Part print with two shaded views. Sizes in mm from the minimum x, y, z corner. Coordinates: 2 decimals unless noted, no trailing zeros. Write each loop counter-clockwise with the first axis right and the second up, starting at its lowest first coordinate (ties: lowest second). Pieces come first, ordered by that corner, then holes. Notation, with made-up numbers: (-4.75, 4.5) - (44.25, 4.5) arc R22 ccw to (44.25, 27.5) - close; hole circle Ø11 at (62.25, -37). An arc over 180 degrees is marked (long way). Answer in a Markdown table with one row per item. Add a question column.
Q1. Pin check, flat tips, straight feed: pin 1 (1 mm diameter, centred on y = 28.5, z = 24.5, fed in from -X); pin 2 (1.5 mm diameter, centred on x = 21, z = 88.5, fed in from -Y); pin 3 (3 mm diameter, centred on y = 28.5, z = 15.5, fed in from +X); pin 4 (10 mm diameter, centred on x = 13, z = 60, fed in from +Y). Stop position of each tip, or through.
Q2. Band-saw the part on C-C (z = 28.5). List the corners of the cut face in (x, y).
Q3. Drill centre lines: line 1 along Y through (x, z) = (15.25, 91.5); line 2 along Y through (x, z) = (15.75, 52.5); line 3 along Z through (x, y) = (13.5, 27.75). Where is each one in solid material? Low to high. Write a range as from..to.
Q4. Band-saw the part on A-A (x = 15). List the corners of the cut face in (y, z).
Q5. Band-saw the part on B-B (z = 82.5). List the corners of the cut face in (x, y), and give its area (3 significant figures).
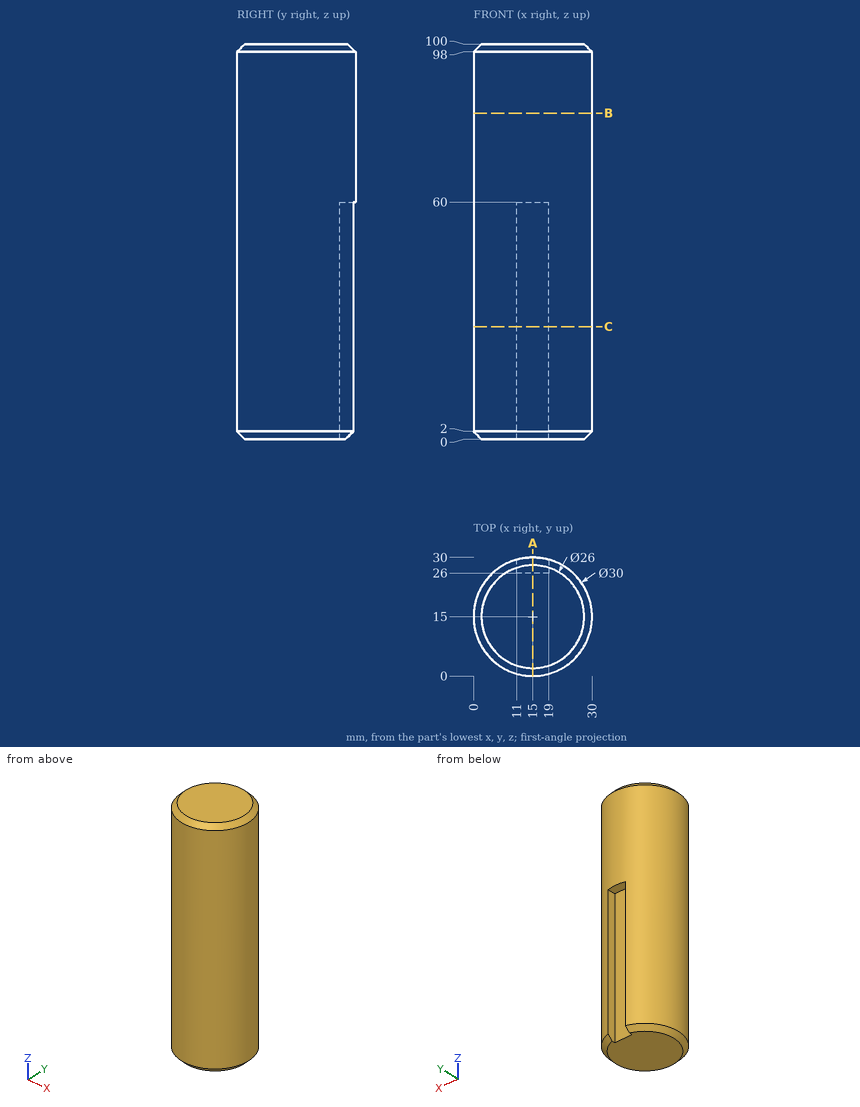
Checked values:
| question | item | result |
|---|---|---|
| 1 | pin 1 | stops at x = 7.52 |
| 1 | pin 2 | stops at y = 0.95 |
| 1 | pin 3 | stops at x = 24 |
| 1 | pin 4 | stops at y = 30 |
| 2 | outline | (11, 26) - (11, 29.46) arc R15 ccw (long way) to (19, 29.46) - (19, 26) - close |
| 3 | line 1 | y = 0..30 |
| 3 | line 2 | y = 0.02..26 |
| 3 | line 3 | z = 60..100 |
| 4 | outline | (0, 2) - (2, 0) - (26, 0) - (26, 60) - (30, 60) - (30, 98) - (28, 100) - (2, 100) - (0, 98) - close |
| 5 | outline | circle Ø30 at (15, 15) |
| 5 | area | 707 mm² |
